from build123d import *

# Parameters (mm, degrees)
SKETCH1_R           = 10
BOSS_EXTRUDE1_DEPTH = 2
SKETCH2_R           = 4.5
BOSS_EXTRUDE2_DEPTH = 2.5
FILLET1_R           = 0.25
SKETCH6_R           = 1
CUT_EXTRUDE2_DEPTH  = 15.840822214
SKETCH7_R           = 2.9
CUT_EXTRUDE3_DEPTH  = 2.5
BOSS_EXTRUDE4_DEPTH = 2.5
CIRPATTERN1_COUNT   = 26
SKETCH3_R           = 1.6
CUT_EXTRUDE4_DEPTH  = 15.361406756
SKETCH9_R           = 3.25
CUT_EXTRUDE5_DEPTH  = 2.6


with BuildPart() as part:
    # Sketch1 → Boss-Extrude1 (new body)
    with BuildSketch(Plane(origin=(0, 0, 0), x_dir=(1, 0, 0), z_dir=(0, 1, 0))):
        with Locations(Location((0, 0, 0), (0, 0, 270))):
            Circle(SKETCH1_R)
    extrude(amount=BOSS_EXTRUDE1_DEPTH)

    # Sketch2 → Boss-Extrude2 (add)
    with BuildSketch(Plane(origin=(0, 0, 0), x_dir=(1, 0, 0), z_dir=(0, 1, 0))):
        with Locations(Location((0, 0, 0), (0, 0, 270))):
            Circle(SKETCH2_R)
    extrude(amount=-BOSS_EXTRUDE2_DEPTH)

    # Fillet1
    fillet1_edges = [part.edges().sort_by_distance(p)[0] for p in [
        (0, 0, -10),
    ]]
    fillet(fillet1_edges, radius=FILLET1_R)

    # Sketch6 → Cut-Extrude2 (cut, through all)
    with BuildSketch(Plane(origin=(0, 2, 0), x_dir=(1, 0, 0), z_dir=(0, 1, 0))):
        with Locations(Location((0, 0, 0), (0, 0, 270))):
            Circle(SKETCH6_R)
    extrude(amount=-CUT_EXTRUDE2_DEPTH, mode=Mode.SUBTRACT)

    # Sketch7 → Cut-Extrude3 (cut)
    with BuildSketch(Plane.XZ.offset(2.5)):
        with Locations(Location((0, 0, 0), (0, 0, 270))):
            Circle(SKETCH7_R)
    extrude(amount=-CUT_EXTRUDE3_DEPTH, mode=Mode.SUBTRACT)

    # Sketch8 → Boss-Extrude4 (add)
    with BuildSketch(Plane.XZ.offset(2.5)):
        with BuildLine():
            Line((-2.35244742, -1.046531787), (-2.745588284, -0.933672842))
            ThreePointArc((-2.745588284, -0.933672842), (-2.649635472, -1.178741646), (-2.531859978, -1.414102207))
            Line((-2.531859978, -1.414102207), (-2.35244742, -1.046531787))
        make_face()
    boss_extrude4 = extrude(amount=-BOSS_EXTRUDE4_DEPTH)

    # CirPattern1: Boss-Extrude4 ×26 about axis
    cirpattern1_axis = Axis((0, 0, 0), (0, 1, 0))
    for i in range(1, CIRPATTERN1_COUNT):
        add(boss_extrude4.rotate(cirpattern1_axis, i * 360 / CIRPATTERN1_COUNT))

    # Sketch3 → Cut-Extrude4 (cut, through all)
    with BuildSketch(Plane(origin=(0, 0, 0), x_dir=(1, 0, 0), z_dir=(0, 1, 0))):
        with Locations(Location((0, 7, 0), (0, 0, 270))):
            Circle(SKETCH3_R)
        with Locations(Location((-7, 0, 0), (0, 0, 270))):
            Circle(SKETCH3_R)
        with Locations(Location((0, -7, 0), (0, 0, 90))):
            Circle(SKETCH3_R)
        with Locations(Location((7, 0, 0), (0, 0, 90))):
            Circle(SKETCH3_R)
    extrude(amount=CUT_EXTRUDE4_DEPTH, mode=Mode.SUBTRACT)

    # Sketch9 → Cut-Extrude5 (cut)
    with BuildSketch(Plane.XZ.offset(2.5)):
        with Locations((7, 0)):
            Circle(SKETCH9_R)
        with Locations((0, -7)):
            Circle(SKETCH9_R)
        with Locations((-7, 0)):
            Circle(SKETCH9_R)
        with Locations((0, 7)):
            Circle(SKETCH9_R)
    extrude(amount=-CUT_EXTRUDE5_DEPTH, mode=Mode.SUBTRACT)


solid = part.part
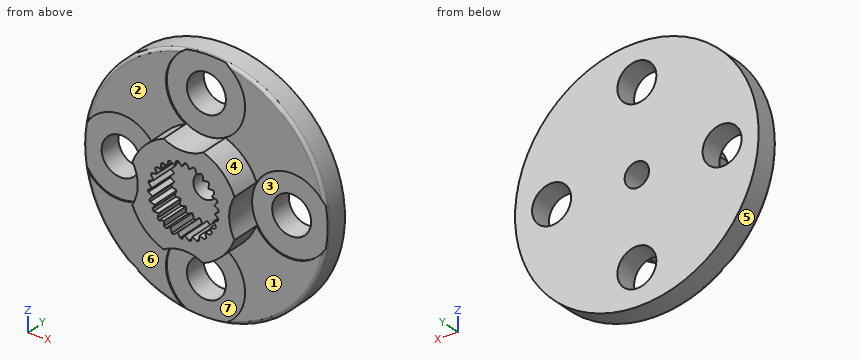
Check sheet for the modelled part. Datum: model origin and axes. Units: mm. Face numbers are marked on the shaded views. A direction names the side the tool comes from. Give positions to 0.01 mm unless a question says otherwise; leave off trailing zeros. Loops run counter-clockwise (first coordinate to the right, second up) from the corner with the lowest first, then second, coordinate; pieces in that order, holes last. Notation, with made-up numbers: M 69,55 L 104,55 A19 cw 104,85 Z; hole C 58.5,-13.5 d11. An arc over 180 degrees is marked long. Return JSON: item names as keys, results as strings. Group by question number.
1. Cross-section at A-A on y = 1.3. Record the boundary of the cut face in (x, z).
2. Tool access check on the marked faces 1, 2, 3 and 4. Record the directions out of +Z, -Z, +X, -X, +Y, -Y that give a thin tool (end or side, any length) a straight path to the whole face; none if there is none.
3. Mould release check, pull along Z, two halves, no side actions. Record for the marked faces 5, 6 and 7: released by +Z, released by -Z, zero draft, split by the parting line, or undercut.
4. Thickness scan on L1, parallel to Y at x = 5, z = 8; L2, parallel to Y at x = -5.75, z = 1.25; L3, parallel to Z at x = 0, y = -0.95. Record the ranges inside material, lowest first.
5. Go/stop test with flat-tipped pins: pin 1 (1.9 mm diameter, centred on x = -8, z = 0, fed in from -Y); pin 2 (1 mm diameter, centred on x = 3.5, y = 1, fed in from -Z). Record where each tip stops, or that it passes through.
Return value:
{
 "1": {"outline": "C 0,0 d20; hole C -7,0 d3.2; hole C 0,-7 d3.2; hole C 0,7 d3.2; hole C 0,0 d2; hole C 7,0 d3.2"},
 "2": {"face 1": "-Z, +X, -Y", "face 2": "+Z, -X, -Y", "face 3": "-Y", "face 4": "+Z, +X, -Y"},
 "3": {"face 5": "split by the parting line", "face 6": "zero draft", "face 7": "undercut"},
 "4": {"L1": "0 to 2", "L2": "0.1 to 2", "L3": "-3.75 to -2.76, 2.76 to 3.75"},
 "5": {"pin 1": "y = 0.1", "pin 2": "z = -9.54"}
}
